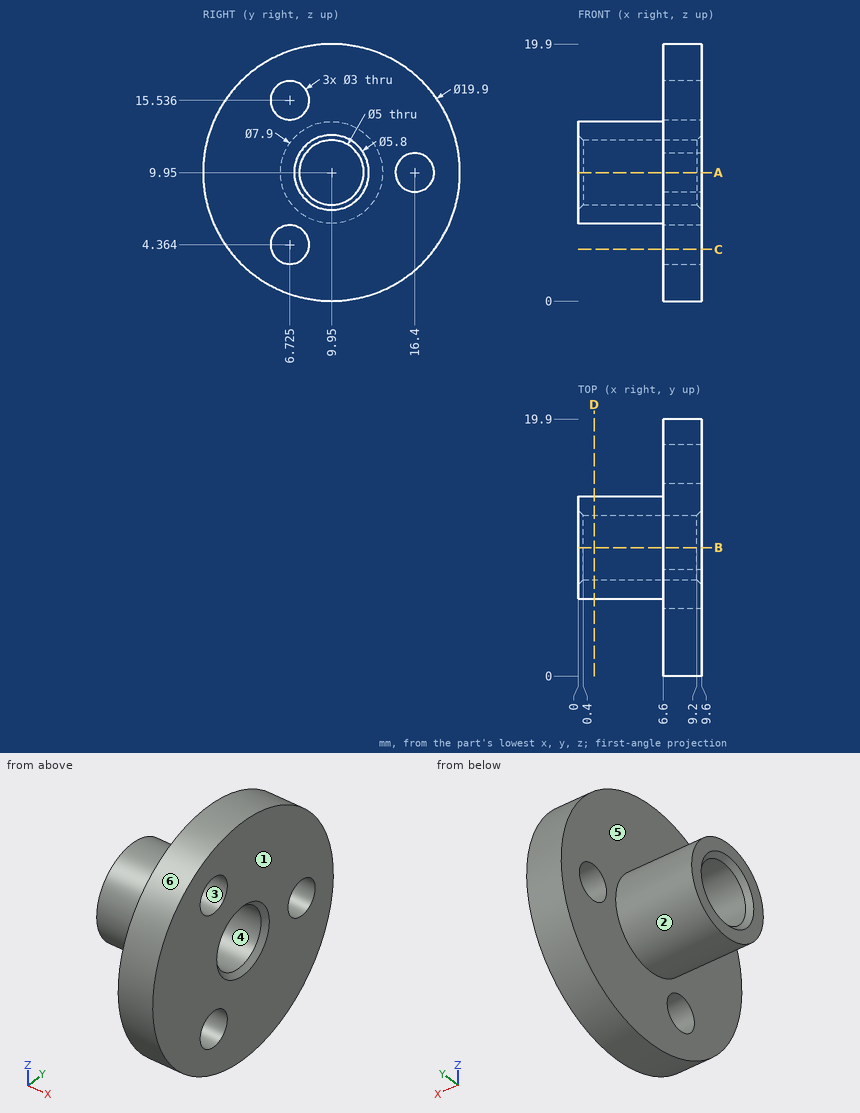
Here's the drawing with two shaded views (mm, measured from the low corner). I have some questions. A direction names the side the tool comes from. Coordinates: 2 decimals unless noted, no trailing zeros. Write each loop counter-clockwise with the first axis right and the second up, starting at its lowest first coordinate (ties: lowest second). Pieces come first, ordered by that corner, then holes. Notation, with made-up numbers: M -17,16.25 L 5,16.25 A24 ccw 5,49.25 Z; hole C 73,20 d7. An arc over 180 degrees is marked long. Answer as CSV lines item,"result".
Item 1: On a 3-axis mill with a long thin cutter (end or side, diameter ignored), from which of +Z, -Z, +X, -X, +Y, -Y can I reach the whole of each face in a straight line? I mean the marked faces 5 and 6. Say none if no direction works.
Geometry results:
face 5,"-X"
face 6,"+X, -X"
Item 2: Imagine slicing it at B-B on y = 9.95. List the corners of the cut face in (x, z) for me, plus the area to 3 significant figures.
Geometry results:
outline,"M 0,6 L 6.6,6 L 6.6,0 L 9.6,0 L 9.6,7.05 L 9.2,7.45 L 0.4,7.45 L 0,7.05 Z; M 0,12.85 L 0.4,12.45 L 9.2,12.45 L 9.6,12.85 L 9.6,19.9 L 6.6,19.9 L 6.6,13.9 L 0,13.9 Z"
area,"63.5 mm2"
Item 3: Imagine slicing it at C-C on z = 4. List the corners of the cut face in (x, y) for me (3 decimals).
Geometry results:
outline,"M 6.6,1.975 L 9.6,1.975 L 9.6,5.27 L 6.6,5.27 Z; M 6.6,8.18 L 9.6,8.18 L 9.6,17.925 L 6.6,17.925 Z"
Item 4: Imagine slicing it at D-D on x = 1.25. List the corners of the cut face in (y, z) for me, plus the area to 3 significant figures.
Geometry results:
outline,"C 9.95,9.95 d7.9; hole C 9.95,9.95 d5"
area,"29.4 mm2"
Item 5: Please list where these lines run through material, in increasing order: line 1 along Y through (x, z) = (8, 10); line 2 along Y through (x, z) = (6.5, 9.95); line 3 along X through (y, z) = (5.75, 9.5).
Geometry results:
line 1,"y = 0 to 7.45, 12.45 to 14.9, 17.9 to 19.9"
line 2,"y = 6 to 7.45, 12.45 to 13.9"
line 3,"x = 6.6 to 9.6"
Item 6: I'm going to push flat-ended pins straight in: P1, Ø3, axis at x = 5.5, z = 2.5, coming from the -Y side; P2, Ø5, axis at y = 16.4, z = 9.95, coming from the +X side; P3, Ø4, axis at x = 6, z = 13.5, coming from the +Y side; P4, Ø4, axis at x = 5, y = 4.5, coming from the -Z side. Where does each tip first touch, or does it pass through?
Geometry results:
P1,"stops at y = 2.36"
P2,"stops at x = 9.6"
P3,"stops at y = 19.76"
P4,"stops at z = 0.95"
Item 7: Imagine slicing it at A-A on z = 9.95. List the corners of the cut face in (x, y) for me.
Geometry results:
outline,"M 0,6 L 6.6,6 L 6.6,0 L 9.6,0 L 9.6,7.05 L 9.2,7.45 L 0.4,7.45 L 0,7.05 Z; M 0,12.85 L 0.4,12.45 L 9.2,12.45 L 9.6,12.85 L 9.6,14.9 L 6.6,14.9 L 6.6,13.9 L 0,13.9 Z; M 6.6,17.9 L 9.6,17.9 L 9.6,19.9 L 6.6,19.9 Z"
Item 8: We'd pull the mould along Z, two halves only. Please class the marked faces 1, 2, 3 and 4: +Z half, -Z half, draft (parallel to the pull), parting line (faces both ways), or undercut.
Geometry results:
face 1,"draft"
face 2,"parting line"
face 3,"undercut"
face 4,"undercut"
